Part model, mm, in its own coordinate system. Face numbers are marked on the shaded views. A direction names the side the tool comes from. Give positions to 0.01 mm unless a question says otherwise; leave off trailing zeros. Loops run counter-clockwise (first coordinate to the right, second up) from the corner with the lowest first, then second, coordinate; pieces in that order, holes last. Notation, with made-up numbers: (59, 18) -> (96, 18) arc R20 cw to (96, 38) -> close; hole circle Ø8 at (51, 10). An arc over 180 degrees is marked (long way). One line per question, with ' | ' between items.
```python
from build123d import *

# Parameters (mm, degrees)
SKETCH1_R           = 16
BOSS_EXTRUDE1_DEPTH = 8
CUT_EXTRUDE2_DEPTH  = 5


with BuildPart() as part:
    # Sketch1 → Boss-Extrude1 (new body)
    with BuildSketch(Plane(origin=(0, 0, 0), x_dir=(1, 0, 0), z_dir=(0, 1, 0))):
        with Locations(Location((-62.417227704, 31.446847546, 0), (0, 0, 270))):
            Circle(SKETCH1_R)
    extrude(amount=BOSS_EXTRUDE1_DEPTH)

    # Sketch9 → Cut-Extrude2 (cut)
    with BuildSketch(Plane(origin=(0, 8, 0), x_dir=(1, 0, 0), z_dir=(0, 1, 0))):
        with BuildLine():
            Line((-66.417227704, 41.693798311), (-66.417227704, 31.446847546))
            Line((-66.417227704, 31.446847546), (-66.417227704, 21.19989678))
            add(Edge.make_bspline(
                [(-66.417227704, 41.693798311), (-80.417227704, 31.446847546), (-66.417227704, 21.19989678)],
                knots=[0, 0, 0, 1, 1, 1], degree=2))
        make_face()
        with BuildLine():
            Line((-58.417227704, 41.693798311), (-58.417227704, 21.19989678))
            add(Edge.make_bspline(
                [(-58.417227704, 41.693798311), (-44.417227704, 31.446847546), (-58.417227704, 21.19989678)],
                knots=[0, 0, 0, 1, 1, 1], degree=2))
        make_face()
    extrude(amount=-CUT_EXTRUDE2_DEPTH, mode=Mode.SUBTRACT)


solid = part.part
```
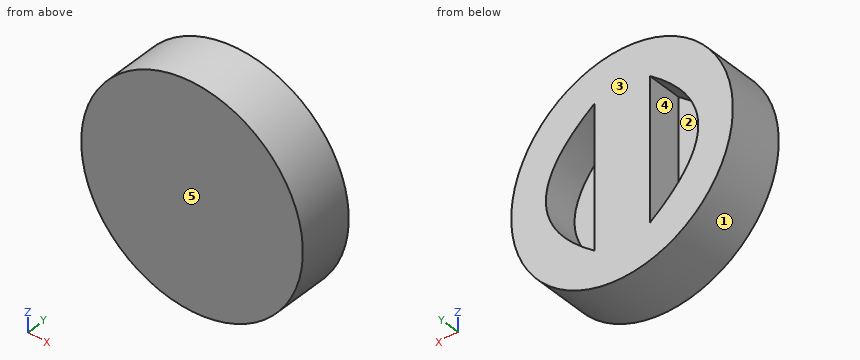
1) Saw through at D-D (y = 4). State how many separate pieces and enclosed holes the cut face has, and give its area (3 significant figures).
Found:
separate pieces: 1 | enclosed holes: 2 | area: 613 mm2
2) Pin check, flat tips, straight feed: P1, Ø1.5, axis at x = -70, y = 1.5, coming from the +Z side; P2, Ø2, axis at y = 5.5, z = -29.5, coming from the -X side; P3, Ø1.5, axis at y = 2.5, z = -20, coming from the +X side. Stop position of each tip, or through.
Found:
P1: z = -16.98 | P2: x = -78.39 | P3: x = -50.52
3) Saw through at A-A (y = 1). Give the cut face in (x, z).
Found:
outline: circle Ø32 at (-62.42, -31.45)
4) Pull direction Z, two halves, no side cores. Call the marked faces 1, 2 and 3: pulls with the +Z half, pulls with the -Z half, needs draft (parallel to the pull), parting line crosses it, or undercut.
Found:
face 1: parting line crosses it | face 2: undercut | face 3: needs draft
5) Saw through at B-B (z = -43). Give the cut face in (x, y), and give its area (3 significant figures).
Found:
outline: (-73.49, 0) -> (-51.35, 0) -> (-51.35, 8) -> (-73.49, 8) -> close | area: 177 mm2
6) Tool access for the marked faces 4 and 5: list every direction of +Z, -Z, +X, -X, +Y, -Y with a clear straight run to the whole face (end or side of a thin tool).
Found:
face 4: +Y | face 5: +Z, -Z, +X, -X, -Y
7) Drill centre lines: line 1 (X direction, y = 3.25, z = -40.5); line 2 (X direction, y = 7, z = -34.5); line 3 (Z direction, x = -69, y = 4.25). Where is each one in solid material? Low to high.
Found:
line 1: -75.61 to -67.95, -66.42 to -58.42, -56.88 to -49.22 | line 2: -78.12 to -72.8, -66.42 to -58.42, -52.04 to -46.71 | line 3: -46.03 to -39.59, -23.31 to -16.86
8) Saw through at C-C (x = -76). Give the cut face in (y, z).
Found:
outline: (0, -39.9) -> (8, -39.9) -> (8, -22.99) -> (0, -22.99) -> close
